Part model, mm, in its own coordinate system. A direction names the side the tool comes from. Give positions to 0.01 mm unless a question says otherwise; leave off trailing zeros. Loops run counter-clockwise (first coordinate to the right, second up) from the corner with the lowest first, then second, coordinate; pieces in that order, holes last. Notation, with made-up numbers: (1, -21.5) -> (23, -21.5) arc R15 ccw to (23, -14.5) -> close; hole circle Ø8 at (-11.75, -22.5). An arc over 180 degrees is marked (long way). Write item = value, one per line.
Autodesk Inventor part; units mm, degrees
ref_plane "YZ Plane" through (0, 0, 0) normal (1, 0, 0) x (0, 1, 0)
ref_plane "XZ Plane" through (0, 0, 0) normal (0, 1, 0) x (-1, 0, 0)
ref_plane "XY Plane" through (0, 0, 0) normal (0, 0, 1) x (1, 0, 0)
sketch "Sketch1" plane through (0, 0, 0) normal (0, 0, 1) x (1, 0, 0)
  line L0 (30, 158) -> (30, 0) construction
  line L1 (0, 0) -> (0, 155)
  line L2 (0, 0) -> (30, 0)
  line L3 (30, 0) -> (0, 0) construction
  line L4 (0, 0) -> (0, 3) construction
  line L5 (0, 3) -> (27, 3)
  line L6 (27, 3) -> (27, 155)
  line L7 (27, 155) -> (0, 155)
  line L8 (0, 155) -> (0, 158)
  line L9 (0, 158) -> (30, 158) construction
  line L10 (27, 158) -> (27, 161) construction
  arc A0 (28.5, 159.5) -> (25.5, 159.5) centre (27, 159.5) ccw
  line L11 (28.5, 159.5) -> (28.5, 158) construction
  line L12 (25.5, 159.5) -> (25.5, 158)
  line L13 (27, 155) -> (27, 158) construction
  arc A1 (28.5, 159.5) -> (29.2857, 157.8283) centre (30.6712, 159.5) ccw
  arc A2 (30, 156.3085) -> (29.2857, 157.8283) centre (28.0261, 156.3085) ccw
  line L14 (25.5, 158) -> (0, 158)
  line L15 (30, 156.3085) -> (30, 0)
  point P0 (30, 79)
  dimension "d0" = 60
  dimension "d1" = 158
  dimension "d2" = 3
  dimension "d3" = 27
  dimension "d4" = 3
  dimension "d5" = 3
  dimension "d6" = 1.5
revolve "Revolution1" add sketch "Sketch1" angle 360 about axis through (0, 0, 0) along (0, 1, 0) contours L1 L5 L6 L7 L8 L14 L12 A0 A1 A2 L15 L2
fillet "Fillet1" radius 2 1 edges at (-30, 0, 0)
sketch "Sketch2" plane through (0, 158, 0) normal (0, 1, 0) x (1, 0, 0)
  circle A0 centre (0, 0) radius 25.5 construction
  circle A1 centre (5.1723, 0) radius 4.542 construction
  circle A2 centre (17.4125, 0) radius 6.2476 construction
  line L0 (4.5394, -4.4977) -> (16.5419, -6.1866)
  line L1 (4.5394, 4.4977) -> (16.5419, 6.1866)
  arc A3 (4.5394, 4.4977) -> (4.5394, -4.4977) centre (5.1723, 0) ccw
  arc A4 (16.5419, -6.1866) -> (16.5419, 6.1866) centre (17.4125, 0) ccw
  circle A5 centre (5.1723, 0) radius 2.3915
  arc A6 (19.1723, 4.25) -> (19.1723, -4.25) centre (22.6879, 0) ccw
  arc A7 (19.1723, -4.25) -> (19.1723, 4.25) centre (15.6567, 0) ccw
  arc A8 (17.8945, -2.7286) -> (20.4501, -2.7286) centre (19.1723, 0.1434) ccw
  arc A9 (20.4501, 2.7286) -> (17.8945, 2.7286) centre (19.1723, -0.1434) ccw
  line L2 (17.8945, -2.7286) -> (17.8945, 2.7286) construction
  line L3 (20.4501, -2.7286) -> (20.4501, 2.7286) construction
  line L4 (17.4125, 0) -> (5.1723, 0) construction
  line L5 (17.1723, 0) -> (21.1723, 0) construction
  point P0 (20.4501, 0)
  point P1 (19.1723, 3)
  point P2 (19.1723, -3)
  dimension "d9" = 12.4952
  dimension "d10" = 9.084
  dimension "d11" = 17.4125
  dimension "d12" = 5.1723
  dimension "d13" = 12.2402
  dimension "d14" = 8.5
  dimension "d15" = 16
  dimension "d16" = 6
  dimension "d17" = 4
  dimension "d18" = 3.1434
  dimension "d19" = 4.783
extrude "Extrusion1" add sketch "Sketch2" along normal blind 2 contours A3 L1 A4 L0 | A7 A9 A6 | A8 A7 A6
properties part number "the cup"
1) Drill centre lines: line 1 along X through (y, z) = (159.6, 0); line 2 along Y through (x, z) = (-4, 17); line 3 along Z through (x, y) = (0, 40.5). Where is each one in solid material? Low to high. Write a range as [from, to].
Resolved:
line_1 = [-28.5, -25.5], [0.63, 2.78], [7.56, 17.17], [21.17, 23.66], [25.5, 28.5]
line_2 = [0, 3], [155, 158]
line_3 = [-30, -27], [27, 30]
2) Drop flat-ended pins along their axis: P1, Ø5, axis at x = 18.5, y = 42.5, coming from the +Z side; P2, Ø1, axis at x = -14, y = 113, coming from the -Z side; P3, Ø16, axis at x = -3.5, z = 12.5, coming from the +Y side; P4, Ø4, axis at x = -10.5, z = -21, coming from the -Y side. Give the stop position or say it passes through.
Resolved:
P1 = 25.38
P2 = -26.79
P3 = 158
P4 = 0
3) Which spindle directions (+Z, -Z, +X, -X, +Y, -Y) get a long thin tool onto all of the face, cutting with end or side? Do faces 5 (the face through (0, 155, 0)), 6 (the face through (-5.5, 158.7, -24.9)). Say none if no direction does.
Resolved:
face_5 = none
face_6 = +Y
4) Slice it at B-B, the plane y = 98. List the corners of the cut face in (x, z), and give its area (3 significant figures).
Resolved:
outline = circle Ø60 at (0, 0); hole circle Ø54 at (0, 0)
area = 537 mm²
5) Pull direction Z, two halves, no side cores. Call faces 1 (the face through (0, 3, 0)), 2 (the face through (0, 0, 0)), 3 (the face through (5, 158, 0)), 4 (the face through (-29.97, 78.07, 1.32)): pulls with the +Z half, pulls with the -Z half, needs draft (parallel to the pull), parting line crosses it, or undercut.
Resolved:
face_1 = undercut
face_2 = needs draft
face_3 = undercut
face_4 = parting line crosses it
